Check sheet for the modelled part. Datum: model origin and axes. Units: mm. A direction names the side the tool comes from. Give positions to 0.01 mm unless a question says otherwise; leave off trailing zeros. Order: outer loops, then holes, each group sorted by start corner. A loop starts at its lowest first (then second) coordinate and runs counter-clockwise, first axis right, second up. Notation, with made-up numbers: (74, 7.5) -> (92, 7.5) arc R38 cw to (92, 45.5) -> close; hole circle Ø5 at (-12.5, 10.5). An arc over 180 degrees is marked (long way). One line per question, with ' | ' between items.
```python
from build123d import *

# Parameters (mm, degrees)
PLACA_SUPERIOR_ACROMION_DEPTH  = 3.5
PLACA_POSTERIOR_ESCAPULA_DEPTH = 3.5
SKETCH3_W                      = 140
SKETCH3_H                      = 64
PLACA_ANTERIOR_DEPTH           = 3.5
SKETCH4_W                      = 22
SKETCH4_H                      = 20
CUELLO_GLENOIDEO_DEPTH         = 54
SKETCH6_W                      = 120
SKETCH6_H                      = 56
VENTANA_POSTERIOR_DEPTH        = 6
SKETCH7_W                      = 100
SKETCH7_H                      = 26
VENTANA_ANTERIOR_DEPTH         = 6


with BuildPart() as part:
    # Sketch1 → Placa_superior_acromion (new body)
    with BuildSketch(Plane(origin=(0, 38.5, 0), x_dir=(1, 0, 0), z_dir=(0, 1, 0))):
        Polygon((-172, -60), (16, -60), (36, -18), (36, 18), (16, 60), (-172, 60), align=None)
    extrude(amount=PLACA_SUPERIOR_ACROMION_DEPTH)

    # Sketch2 → Placa_posterior_escapula (add)
    with BuildSketch(Plane.XY.offset(26.5)):
        Polygon((-172, 40), (-10, 40), (-10, -22), (-22, -86), (-172, -86), align=None)
    extrude(amount=PLACA_POSTERIOR_ESCAPULA_DEPTH)

    # Sketch3 → Placa_anterior (add)
    with BuildSketch(Plane.XY.offset(-30)):
        with Locations((-80, 8)):
            Rectangle(SKETCH3_W, SKETCH3_H)
    extrude(amount=PLACA_ANTERIOR_DEPTH)

    # Sketch4 → Cuello_glenoideo (add)
    with BuildSketch(Plane.XY.offset(-27)):
        with Locations((-25, 30)):
            Rectangle(SKETCH4_W, SKETCH4_H)
    extrude(amount=CUELLO_GLENOIDEO_DEPTH)

    # Sketch5 → Cavidad_glenoidea (revolve)
    with BuildSketch(Plane.XY, mode=Mode.PRIVATE) as cavidad_glenoidea_sk:
        Polygon((-36, 0), (-36, 27.5), (-12, 27.5), (-11.77481768, 19.290248018), (-15.980613255, 15.980613255), (-19.572174126, 11.3), (-21.829923674, 5.849310419), (-22.6, 0), align=None)
    revolve(cavidad_glenoidea_sk.sketch.rotate(Axis((-40, 0, 0), (1, 0, 0)), 90), axis=Axis((-40, 0, 0), (1, 0, 0)))

    # Sketch6 → Ventana_posterior (cut)
    with BuildSketch(Plane.XY.offset(25)):
        with Locations((-100, -6)):
            Rectangle(SKETCH6_W, SKETCH6_H)
    extrude(amount=VENTANA_POSTERIOR_DEPTH, mode=Mode.SUBTRACT)

    # Sketch7 → Ventana_anterior (cut)
    with BuildSketch(Plane.XY.offset(-31)):
        with Locations((-90, -3)):
            Rectangle(SKETCH7_W, SKETCH7_H)
    extrude(amount=VENTANA_ANTERIOR_DEPTH, mode=Mode.SUBTRACT)


solid = part.part
```
Q1. Mould release check, pull along Z, two halves, no side actions. Record for faces 5 (the face through (26, 40, 39)), 6 (the face through (26, 40, -39)), 7 (the face through (-69, 38.5, -1)), 8 (the face through (-172, 39, 0)): pulls with the +Z half, pulls with the -Z half, needs draft (parallel to the pull), parting line crosses it, or undercut.
Result sheet:
face 5: pulls with the +Z half | face 6: pulls with the -Z half | face 7: undercut | face 8: needs draft
Q2. Thickness scan on line 1 (Y direction, x = -114, z = 15); line 2 (Z direction, x = -23, y = 16); line 3 (Z direction, x = -142, y = 13.5). Record the ranges inside material, lowest first.
Result sheet:
line 1: y = 38.5 to 42 | line 2: z = -30 to -26.5, -22.37 to 22.37, 26.5 to 30 | line 3: z = -30 to -26.5
Q3. Section check D-D (x = 4.5). Enter the section's corners in (y, z), and give its area (3 significant figures).
Result sheet:
outline: (38.5, -60) -> (42, -60) -> (42, 60) -> (38.5, 60) -> close | area: 420 mm2
Q4. Section check B-B (x = -45.5). Enter the section's corners in (y, z).
Result sheet:
outline: (-86, 26.5) -> (-34, 26.5) -> (-34, 30) -> (-86, 30) -> close; (-24, -30) -> (-16, -30) -> (-16, -26.5) -> (-24, -26.5) -> close; (10, -30) -> (38.5, -30) -> (38.5, -60) -> (42, -60) -> (42, 60) -> (38.5, 60) -> (38.5, 30) -> (22, 30) -> (22, 26.5) -> (38.5, 26.5) -> (38.5, -26.5) -> (10, -26.5) -> close
Q5. Access from +Z, -Z, +X, -X, +Y, -Y to the whole of each face (thin tool, end or side, straight path). Record for faces 1 (the face through (-81, 15, -30)), 2 (the face through (-69, 42, -1)), 3 (the face through (-36, 5, 0)), 4 (the face through (-14, 31, 0)).
Result sheet:
face 1: -Z, +X, -X, -Y | face 2: +Z, -Z, +X, -X, +Y | face 3: -X, -Y | face 4: +X
Q6. Section check C-C (y = -74). Enter the section's corners in (x, z), and give its area (3 significant figures).
Result sheet:
outline: (-172, 26.5) -> (-19.75, 26.5) -> (-19.75, 30) -> (-172, 30) -> close | area: 533 mm2
Q7. Depth check by flat-ended pin: pin 1 Ø1 at (y, z) = (-1.5, -28.5) entering from +X; pin 2 Ø2 at (x, y) = (-13, -40.5) entering from +Z; pin 3 Ø3 at (x, y) = (-88, -66.5) entering from -Z. Enter the tip coordinate at first touch or a pass-through.
Result sheet:
pin 1: stops at x = -10 | pin 2: stops at z = 30 | pin 3: stops at z = 26.5
Q8. Section check A-A (x = -153). Enter the section's corners in (y, z), and give its area (3 significant figures).
Result sheet:
outline: (-86, 26.5) -> (-34, 26.5) -> (-34, 30) -> (-86, 30) -> close; (22, 26.5) -> (38.5, 26.5) -> (38.5, -60) -> (42, -60) -> (42, 60) -> (38.5, 60) -> (38.5, 30) -> (22, 30) -> close | area: 660 mm2
